```python
from build123d import *

# Parameters (mm, degrees)
SKETCH1_W           = 157.185890266
SKETCH1_H           = 76.388087763
BOSS_EXTRUDE1_DEPTH = 30
SKETCH2_R           = 4
SKETCH2_R_2         = 16.751919573
CUT_EXTRUDE1_DEPTH  = 8
BOSS_EXTRUDE5_DEPTH = 8
SKETCH8_R           = 0.7
BOSS_EXTRUDE6_DEPTH = 1


with BuildPart() as part:
    # Sketch1 → Boss-Extrude1 (new body)
    with BuildSketch(Plane(origin=(0, 0, 0), x_dir=(1, 0, 0), z_dir=(0, 1, 0))):
        with Locations((-65.664274203, 22.88675236)):
            Rectangle(SKETCH1_W, SKETCH1_H)
    extrude(amount=BOSS_EXTRUDE1_DEPTH)

    # Sketch2 → Cut-Extrude1 (cut)
    with BuildSketch(Plane(origin=(0, 30, 0), x_dir=(1, 0, 0), z_dir=(0, 1, 0))):
        with Locations(Location((2.020364903, 24.483023403, 0), (0, 0, 270))):
            Circle(SKETCH2_R)
        with Locations(Location((-12.582950978, 31.07817581, 0), (0, 0, 270))):
            Circle(SKETCH2_R)
        with Locations(Location((-24.034725928, 38.939278582, 0), (0, 0, 270))):
            Circle(SKETCH2_R)
        with Locations(Location((-31.0292801, 49.329254707, 0), (0, 0, 270))):
            Circle(SKETCH2_R)
        with Locations(Location((4.005067314, 41.454528732, 0), (0, 0, 270))):
            Circle(SKETCH2_R)
        with Locations(Location((-77.650582925, 24.483023403, 0), (0, 0, 270))):
            Circle(SKETCH2_R_2)
    extrude(amount=-CUT_EXTRUDE1_DEPTH, mode=Mode.SUBTRACT)

    # Sketch3 → Boss-Extrude5 (add)
    with BuildSketch(Plane(origin=(0, 30, 0), x_dir=(1, 0, 0), z_dir=(0, 1, 0))):
        with BuildLine():
            Line((-115.629013378, 7.30264293), (-131.71869807, 7.30264293))
            ThreePointArc((-131.71869807, 7.30264293), (-136.882446407, 5.163748337), (-139.021341, 0))
            Line((-139.021341, 0), (-108.326370448, 0))
            ThreePointArc((-108.326370448, 0), (-110.465265042, 5.163748337), (-115.629013378, 7.30264293))
        make_face()
    extrude(amount=BOSS_EXTRUDE5_DEPTH)

    # Sketch8 → Boss-Extrude6 (add)
    with BuildSketch(Plane.XY):
        with Locations(Location((-133.40757623, 34.255602161, 0), (0, 0, 180))):
            Circle(SKETCH8_R)
        with Locations(Location((-129.880481724, 34.255602161, 0), (0, 0, 180))):
            Circle(SKETCH8_R)
        with Locations(Location((-126.621646944, 34.255602161, 0), (0, 0, 180))):
            Circle(SKETCH8_R)
        with Locations(Location((-122.826292713, 34.255602161, 0), (0, 0, 180))):
            Circle(SKETCH8_R)
        with Locations(Location((-118.643776602, 34.255602161, 0), (0, 0, 180))):
            Circle(SKETCH8_R)
        with Locations(Location((-114.360631583, 34.255602161, 0), (0, 0, 180))):
            Circle(SKETCH8_R)
    extrude(amount=BOSS_EXTRUDE6_DEPTH)


solid = part.part
```
The listing builds one solid part. Answer for the finished solid, in the listing's coordinates (mm). A direction names the side the tool comes from. Give positions to 0.01 mm unless a question says otherwise; leave off trailing zeros. Order: outer loops, then holes, each group sorted by start corner. A loop starts at its lowest first (then second) coordinate and runs counter-clockwise, first axis right, second up. Notation, with made-up numbers: M 4.25,-32 L 29.25,-32 A15 cw 29.25,-27 Z; hole C 29.25,34 d10. An arc over 180 degrees is marked long. Put each result on its own line as item: value. Start each with the question number.
Item 1: The part is cut by section C-C, the plane z = 9.5. Determine the outline of the cut face in (x, y).
Item 2: The part is cut by section B-B, the plane z = -51. Determine the outline of the cut face in (x, y), and give its area (3 significant figures).
Item 3: Find the intervals of material crossed by line 1 along Y through (x, z) = (-31.5, -31.5); line 2 along Y through (x, z) = (-10, -32); line 3 along Z through (x, y) = (-76, 23), in increasing order.
Item 4: The part is cut by section D-D, the plane z = -2. Determine the outline of the cut face in (x, y), and give its area (3 significant figures).
Item 5: The part is cut by section A-A, the plane y = 27. Determine the outline of the cut face in (x, z).
Item 6: Flat-ended cylindrical pins translate along their axes: P1, Ø5, axis at x = -24.03, z = -38.94, coming from the +Y side; P2, Ø4, axis at x = -32.5, z = -51, coming from the +Y side; P3, Ø4, axis at x = -129.5, y = 36, coming from the +Z side. Find the tip coordinate at first contact, or state that the pin passes through.
Item 7: Which of the six approach directions +Z, -Z, +X, -X, +Y, -Y give full straight-line access (tool end or side, diameter ignored) to faces 5 (the face through (-144.257, 15, -22)), 6 (the face through (-110.4, 33.9, -5.1)), 7 (the face through (-124, 38, -4)), 8 (the face through (-124, 34, -7.303)), 9 (the face through (0.488, 26.056, -20.788))?
Item 8: For a pull along Z with two mould halves and no side action, classify faces 1 (the face through (5.21, 26.06, -37.64)), 2 (the face through (-67, 30, -6)), 3 (the face through (-67, 15, -61.081)), 4 (the face through (-67, 15, 15.307)) as +Z half, -Z half, draft (parallel to the pull), parting line (faces both ways), or undercut.
Answer key:
1. outline: M -144.26,0 L 12.93,0 L 12.93,30 L -144.26,30 Z
2. outline: M -144.26,0 L 12.93,0 L 12.93,30 L -27.39,30 L -27.39,22 L -34.66,22 L -34.66,30 L -144.26,30 Z
2. area: 4,660 mm²
3. line 1: y = 0 to 30
3. line 2: y = 0 to 22
3. line 3: z = -61.08 to -41.15, -7.81 to 15.31
4. outline: M -144.26,0 L 12.93,0 L 12.93,30 L -108.61,30 L -108.61,38 L -138.74,38 L -138.74,30 L -144.26,30 Z
4. area: 4,960 mm²
5. outline: M -144.26,-61.08 L 12.93,-61.08 L 12.93,15.31 L -144.26,15.31 Z; hole C -77.65,-24.48 d33.5; hole C -31.03,-49.33 d8; hole C -24.03,-38.94 d8; hole C -12.58,-31.08 d8; hole C 2.02,-24.48 d8; hole C 4.01,-41.45 d8
6. P1: stops at y = 22
6. P2: stops at y = 30
6. P3: stops at z = 1
7. face 5: +Z, -Z, -X, +Y, -Y
7. face 6: -Z, +X, +Y
7. face 7: +Z, -Z, +X, -X, +Y
7. face 8: -Z, +X, -X, +Y
7. face 9: +Y
8. face 1: undercut
8. face 2: draft
8. face 3: -Z half
8. face 4: +Z half
